from build123d import *

# Parameters (mm, degrees)
SKETCH1_W           = 49.022
SKETCH1_H           = 18.6944
SKETCH1_W_2         = 38.1
SKETCH1_H_2         = 1.5875
BOSS_EXTRUDE1_DEPTH = 1.5875
CUT_EXTRUDE1_REACH  = 53.735
FILLET1_R           = 0.254
FILLET2_R           = 1.27


with BuildPart() as part:
    # Sketch1 → Boss-Extrude1 (new body)
    # profile 1 of 2: a face of its own
    with BuildSketch(Plane.XY.offset(56.947143149)):
        with Locations((11.232994638, 28.020399012)):
            Rectangle(SKETCH1_W, SKETCH1_H)
        Polygon((-11.881005362, 20.959199012), (-11.881005362, 22.546699012), (-10.992005362, 22.546699012), (-8.706005362, 22.546699012), (-7.817005362, 22.546699012), (-7.817005362, 20.959199012), (-8.706005362, 20.959199012), (-10.992005362, 20.959199012), align=None, mode=Mode.SUBTRACT)
        Polygon((33.457994638, 22.546699012), (34.346994638, 22.546699012), (34.346994638, 20.959199012), (33.457994638, 20.959199012), (31.171994638, 20.959199012), (30.282994638, 20.959199012), (30.282994638, 22.546699012), (31.171994638, 22.546699012), align=None, mode=Mode.SUBTRACT)
        Polygon((31.171994638, 33.494099012), (30.282994638, 33.494099012), (-7.817005362, 33.494099012), (-8.706005362, 33.494099012), (-10.992005362, 33.494099012), (-11.881005362, 33.494099012), (-11.881005362, 35.081599012), (-10.992005362, 35.081599012), (-8.706005362, 35.081599012), (-7.817005362, 35.081599012), (30.282994638, 35.081599012), (31.171994638, 35.081599012), (33.457994638, 35.081599012), (34.346994638, 35.081599012), (34.346994638, 33.494099012), (33.457994638, 33.494099012), align=None, mode=Mode.SUBTRACT)
    # profile 2 of 2: a face of its own
    with BuildSketch(Plane.XY.offset(56.947143149)):
        with Locations((11.232994638, 34.287849012)):
            Rectangle(SKETCH1_W_2, SKETCH1_H_2)
    extrude(amount=BOSS_EXTRUDE1_DEPTH)

    # Sketch3 → Cut-Extrude1 (cut, up to next)
    with BuildSketch(Plane.XY.offset(58.534643149), mode=Mode.PRIVATE) as cut_extrude1_sk1:
        Polygon((11.232994638, 25.734399012), (-4.006890486, 20.959199012), (26.472879762, 20.959199012), align=None)
    cut_extrude1_tool1 = extrude(cut_extrude1_sk1.sketch, amount=-CUT_EXTRUDE1_REACH, mode=Mode.PRIVATE) & part.part
    # Sketch3 → Cut-Extrude1 (cut, up to next)
    with BuildSketch(Plane.XY.offset(58.534643149), mode=Mode.PRIVATE) as cut_extrude1_sk2:
        Polygon((13.518994638, 28.020399012), (26.472879762, 31.208099012), (33.457994638, 31.208099012), (33.457994638, 24.832699012), (26.472879762, 24.832699012), align=None)
    cut_extrude1_tool2 = extrude(cut_extrude1_sk2.sketch, amount=-CUT_EXTRUDE1_REACH, mode=Mode.PRIVATE) & part.part
    # Sketch3 → Cut-Extrude1 (cut, up to next)
    with BuildSketch(Plane.XY.offset(58.534643149), mode=Mode.PRIVATE) as cut_extrude1_sk3:
        Polygon((11.232994638, 30.306399012), (-4.006890486, 35.081599012), (26.472879762, 35.081599012), align=None)
    cut_extrude1_tool3 = extrude(cut_extrude1_sk3.sketch, amount=-CUT_EXTRUDE1_REACH, mode=Mode.PRIVATE) & part.part
    # Sketch3 → Cut-Extrude1 (cut, up to next)
    with BuildSketch(Plane.XY.offset(58.534643149), mode=Mode.PRIVATE) as cut_extrude1_sk4:
        Polygon((-4.006890486, 31.208099012), (-10.992005362, 31.208099012), (-10.992005362, 24.832699012), (-4.006890486, 24.832699012), (8.946994638, 28.020399012), align=None)
    cut_extrude1_tool4 = extrude(cut_extrude1_sk4.sketch, amount=-CUT_EXTRUDE1_REACH, mode=Mode.PRIVATE) & part.part
    add(cut_extrude1_tool1.solids().sort_by_distance((11.232995, 22.550932, 58.534643))[0], mode=Mode.SUBTRACT)
    add(cut_extrude1_tool2.solids().sort_by_distance((26.207595, 28.020399, 58.534643))[0], mode=Mode.SUBTRACT)
    add(cut_extrude1_tool3.solids().sort_by_distance((11.232995, 33.489866, 58.534643))[0], mode=Mode.SUBTRACT)
    add(cut_extrude1_tool4.solids().sort_by_distance((-3.741606, 28.020399, 58.534643))[0], mode=Mode.SUBTRACT)

    # Fillet1
    fillet1_edges = [part.edges().sort_by_distance(p)[0] for p in [
        (-4.006890486, 35.081599012, 57.740893149),
        (26.472879762, 35.081599012, 57.740893149),
        (8.946994638, 28.020399012, 57.740893149),
        (-4.006890486, 20.959199012, 57.740893149),
        (26.472879762, 20.959199012, 57.740893149),
        (13.518994638, 28.020399012, 57.740893149),
    ]]
    fillet(fillet1_edges, radius=FILLET1_R)

    # Fillet2
    fillet2_edges = [part.edges().sort_by_distance(p)[0] for p in [
        (-10.992005362, 31.208099012, 57.740893149),
        (-10.992005362, 24.832699012, 57.740893149),
        (-13.278005362, 37.367599012, 57.740893149),
        (35.743994638, 37.367599012, 57.740893149),
        (35.743994638, 18.673199012, 57.740893149),
        (-13.278005362, 18.673199012, 57.740893149),
        (33.457994638, 31.208099012, 57.740893149),
        (33.457994638, 24.832699012, 57.740893149),
    ]]
    fillet(fillet2_edges, radius=FILLET2_R)


solid = part.part
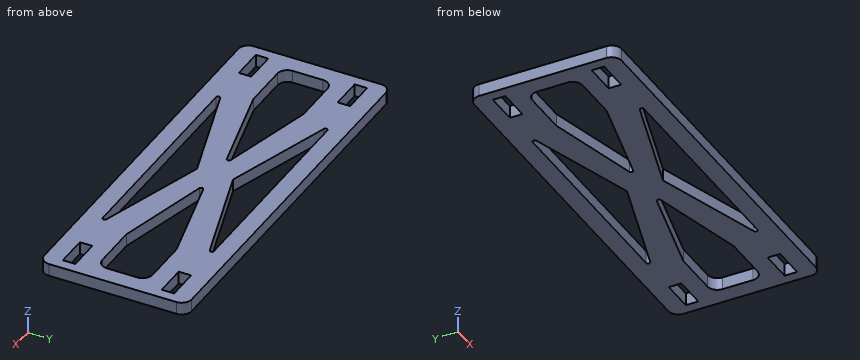
Could you check a few things on this model? Use its own coordinates, in mm. Give positions to 0.01 mm unless a question says otherwise; leave off trailing zeros. Write each loop counter-clockwise with the first axis right and the second up, starting at its lowest first coordinate (ties: lowest second). Pieces come first, ordered by that corner, then holes. Notation, with made-up numbers: (-8.75, -1) -> (3.25, -1) arc R18 ccw to (3.25, 33) -> close; hole circle Ø4 at (-18.75, -18.75). An arc over 180 degrees is marked (long way). Write each question's results on one line, items separated by ' | '. Start each with the question number.
Q1. I need wall thicknesses on probe 1 along Y at (x, z) = (31.5, 58.4); probe 2 along Y at (x, z) = (33.5, 57.3); probe 3 along Y at (x, z) = (11.5, 58.15). Which ranges of each line are inside material? Lowest first, please.
Q2. Suppose I cut it at B-B, the plane x = 25.5. List the corners of the cut face in (y, z) for me, and give its area (3 significant figures).
Q3. Suppose I cut it at D-D, the plane z = 58.1. State how many separate pieces and enclosed holes the cut face has, and give its area (3 significant figures).
Q4. Suppose I cut it at C-C, the plane y = 32.5. List the corners of the cut face in (x, z) for me, and give its area (3 significant figures).
Q5. Suppose I cut it at A-A, the plane x = 7. List the corners of the cut face in (y, z) for me.
Outcome:
1) probe 1: 18.67 to 20.96, 22.55 to 24.83, 31.21 to 33.49, 35.08 to 37.37 | probe 2: 18.67 to 20.96, 22.55 to 33.49, 35.08 to 37.37 | probe 3: 18.67 to 20.96, 25.65 to 30.39, 35.08 to 37.37
2) outline: (18.67, 56.95) -> (25.07, 56.95) -> (25.07, 58.53) -> (18.67, 58.53) -> close; (30.97, 56.95) -> (37.37, 56.95) -> (37.37, 58.53) -> (30.97, 58.53) -> close | area: 20.3 mm2
3) separate pieces: 1 | enclosed holes: 8 | area: 575 mm2
4) outline: (-13.28, 56.95) -> (4.23, 56.95) -> (4.23, 58.53) -> (-13.28, 58.53) -> close; (18.23, 56.95) -> (35.74, 56.95) -> (35.74, 58.53) -> (18.23, 58.53) -> close | area: 55.6 mm2
5) outline: (18.67, 56.95) -> (20.96, 56.95) -> (20.96, 58.53) -> (18.67, 58.53) -> close; (24.41, 56.95) -> (27.54, 56.95) -> (27.54, 58.53) -> (24.41, 58.53) -> close; (28.5, 56.95) -> (31.63, 56.95) -> (31.63, 58.53) -> (28.5, 58.53) -> close; (35.08, 56.95) -> (37.37, 56.95) -> (37.37, 58.53) -> (35.08, 58.53) -> close
